from build123d import *

# Parameters (mm, degrees)
F0_R     = 12.5
F1_DEPTH = 20
F2_W     = 14.4
F2_H     = 2.4
F3_DEPTH = 5
F4_R     = 12.5
F4_R_2   = 7.5
F5_DEPTH = 15
F6_W     = 11.4
F6_H     = 2.4
F7_DEPTH = 15.001
F8_R     = 2
F9_R     = 1


with BuildPart() as f1:
    # F0 (on Top) → F1 (new body)
    with BuildSketch(Plane.XY):
        Circle(F0_R)
    extrude(amount=F1_DEPTH)

    # F2 (on face) → F3 (cut)
    with BuildSketch(Plane.XY.offset(20)):
        Rectangle(F2_W, F2_H)
    extrude(amount=-F3_DEPTH, mode=Mode.SUBTRACT)

    # F4 (on face) → F5 (cut)
    with BuildSketch(Plane(origin=(0, 0, 0), x_dir=(1, 0, 0), z_dir=(0, 0, -1))):
        Circle(F4_R)
        Circle(F4_R_2, mode=Mode.SUBTRACT)
    extrude(amount=-F5_DEPTH, mode=Mode.SUBTRACT)

    # F6 (on face) → F7 (cut, through all)
    with BuildSketch(Plane.XY.offset(15)):
        Rectangle(F6_W, F6_H)
    extrude(amount=-F7_DEPTH, mode=Mode.SUBTRACT)

    # F8
    f8_edges = [f1.edges().sort_by_distance(p)[0] for p in [
        (-7.5, 0, 15),
    ]]
    fillet(f8_edges, radius=F8_R)

    # F9
    f9_edges = [f1.edges().sort_by_distance(p)[0] for p in [
        (-12.5, 0, 20),
        (-12.5, 0, 15),
        (-7.5, 0, 0),
    ]]
    fillet(f9_edges, radius=F9_R)


solid = f1.part
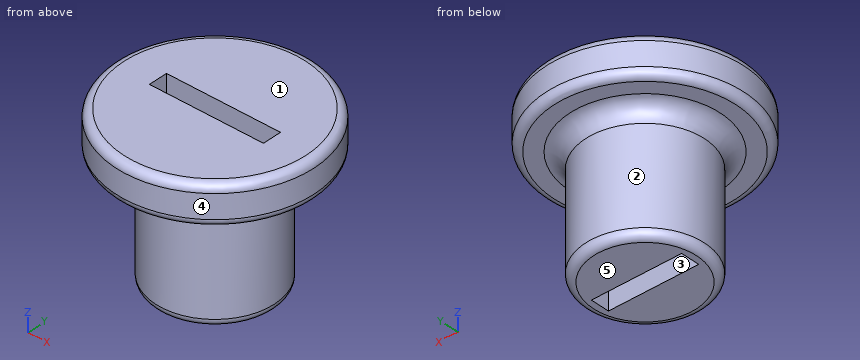
Check sheet for the modelled part. Datum: model origin and axes. Units: mm. Face numbers are marked on the shaded views. A direction names the side the tool comes from. Round coordinates to 2 decimals unless told otherwise and drop trailing zeros. Loops run counter-clockwise (first coordinate to the right, second up) from the corner with the lowest first, then second, coordinate; pieces in that order, holes last. Notation, with made-up numbers: (75, 39) -> (93, 39) arc R16 ccw to (93, 43) -> close; hole circle Ø10 at (21, 22). An arc over 180 degrees is marked (long way). Put each result on its own line as item: value. Start each with the question number.
1. Scan lines: probe 1 along Y at (x, z) = (-3.25, 14.5); probe 2 along Z at (x, y) = (4.25, 10.5); probe 3 along Y at (x, z) = (-4.5, 4.5). Record each from-to range of solid material in increasing order.
2. Section check C-C (z = 10.5). Enter the section's corners in (x, y), plus the area to 3 significant figures.
3. Access from +Z, -Z, +X, -X, +Y, -Y to the whole of each face (thin tool, end or side, straight path). Record for the marked faces 1 and 2.
4. Section check A-A (y = 0). Enter the section's corners in (x, z).
5. Section check D-D (z = 17.5). Enter the section's corners in (x, y).
6. Draft check along Y on the marked faces 3, 4 and 5. Enter one of: +Y half, -Y half, draft (parallel to the pull), parting line (faces both ways), or undercut.
7. Gauge pin test, flat ends, axial feed: pin 1 (1.5 mm diameter, centred on x = -7.5, z = 2, fed in from -Y); pin 2 (2 mm diameter, centred on y = -7, z = 7, fed in from +X); pin 3 (8 mm diameter, centred on x = 9.5, z = 17, fed in from +Y) (3 decimals). Record the tip position at first contact, or that the pin passes through.
8. Section check B-B (x = 0). Enter the section's corners in (y, z).
Findings:
1. probe 1: y = -7.5 to -1.2, 1.2 to 7.5
1. probe 2: z = 15 to 20
1. probe 3: y = -6 to -1.2, 1.2 to 6
2. outline: circle Ø15 at (0, 0); hole (-5.7, -1.2) -> (5.7, -1.2) -> (5.7, 1.2) -> (-5.7, 1.2) -> close
2. area: 149 mm^2
3. face 1: +Z, +X, -X, +Y, -Y
3. face 2: -Z
4. outline: (-12.5, 16) arc R1 ccw to (-11.5, 15) -> (-9.5, 15) arc R2 cw to (-7.5, 13) -> (-7.5, 1) arc R1 ccw to (-6.5, 0) -> (-5.7, 0) -> (-5.7, 15) -> (-7.2, 15) -> (-7.2, 20) -> (-11.5, 20) arc R1 ccw to (-12.5, 19) -> close; (5.7, 0) -> (6.5, 0) arc R1 ccw to (7.5, 1) -> (7.5, 13) arc R2 cw to (9.5, 15) -> (11.5, 15) arc R1 ccw to (12.5, 16) -> (12.5, 19) arc R1 ccw to (11.5, 20) -> (7.2, 20) -> (7.2, 15) -> (5.7, 15) -> close
5. outline: circle Ø25 at (0, 0); hole (-7.2, -1.2) -> (7.2, -1.2) -> (7.2, 1.2) -> (-7.2, 1.2) -> close
6. face 3: undercut
6. face 4: parting line
6. face 5: draft
7. pin 1: stops at y = -3.27
7. pin 2: stops at x = 4.5
7. pin 3: stops at y = 11.225
8. outline: (-12.5, 16) arc R1 ccw to (-11.5, 15) -> (-9.5, 15) arc R2 cw to (-7.5, 13) -> (-7.5, 1) arc R1 ccw to (-6.5, 0) -> (-1.2, 0) -> (-1.2, 20) -> (-11.5, 20) arc R1 ccw to (-12.5, 19) -> close; (1.2, 0) -> (6.5, 0) arc R1 ccw to (7.5, 1) -> (7.5, 13) arc R2 cw to (9.5, 15) -> (11.5, 15) arc R1 ccw to (12.5, 16) -> (12.5, 19) arc R1 ccw to (11.5, 20) -> (1.2, 20) -> close
